Input: part model. Units: mm. Frame: model coordinates. A direction names the side the tool comes from. Give positions to 0.01 mm unless a question says otherwise; leave off trailing zeros. Loops run counter-clockwise (first coordinate to the right, second up) from the corner with the lowest first, then second, coordinate; pieces in that order, holes last. Notation, with made-up numbers: (52.5, 72) - (61.5, 72) arc R36 cw to (61.5, 111) - close; hole circle Ø10 at (-30.5, 20.25). An arc over 180 degrees is marked (long way). Answer as a JSON object with one key per item and string values. Group by question number.
(1) Material intervals for L1, parallel to X at y = -0.4, z = -3; L2, parallel to Y at x = 7.5, z = -7; L3, parallel to Z at x = -2, y = -4.8, sorted ascending.
(2) Section query D-D (z = -4.75). Return loops of the section in (x, y), plus the area to 3 significant figures.
(3) Mould query, pull axis X, two halves, no side actions, for faces 1 (the flat face through (11, -1, -6)), 2 (the flat face through (0, -4, -10)), 3 (the cylindrical face through (-5.55, -0.99, -1.57)). Classes: +X half, -X half, draft (parallel to the pull), parting line (faces both ways), or undercut.
(4) Pin query (flat end, axial travel): P1, Ø2, axis at x = -3, y = -2, coming from the -Z side; P2, Ø2.5, axis at x = 5, y = -4.5, coming from the +Z side; P3, Ø3.5, axis at x = 6, z = -3, coming from the -Y side. Return the tip coordinate at first contact, or that it passes through.
(5) Section query B-B (y = -1.7). Return loops of the section in (x, z), plus the area to 3 significant figures.
(6) Access query for faces 4 (the flat face through (0, -2, -5)), 5 (the cylindrical face through (6.45, -0.99, -1.57)). Directions: +Z, -Z, +X, -X, +Y, -Y. A direction counts if a zero-diameter tool reaches every point of the face in a straight line with its end or side. Return the directions, or none.
(7) Section query C-C (x = 5.75). Return loops of the section in (y, z).
(8) Section query A-A (x = -6). Return loops of the section in (y, z), plus the area to 3 significant figures.
```python
from build123d import *

# Parameters (mm, degrees)
SKETCH1_W                    = 12
SKETCH1_H                    = 2
BASE_FLANGE1_DEPTH           = 11
SKETCH2_R                    = 1.5
CUT_EXTRUDE1_DEPTH           = 10
EDGE_FLANGE1_STRIP_W         = 9.4732
EDGE_FLANGE1_STRIP_H         = 2
EDGE_FLANGE1_STRIP_CUT_DEPTH = 22
EDGE_FLANGE1_DEPTH           = 22


# Sheet-metal steps are written as plain solids
with BuildPart() as part:
    # Sketch1 → Base-Flange1 (new, symmetric)
    with BuildSketch(Plane(origin=(0, 0, 0), x_dir=(0, 0, -1), z_dir=(1, 0, 0))):
        with Locations((6, -1)):
            Rectangle(SKETCH1_W, SKETCH1_H)
    extrude(amount=BASE_FLANGE1_DEPTH, both=True)

    # Sketch2 → Cut-Extrude1 (cut)
    with BuildSketch(Plane(origin=(0, 0, 0), x_dir=(1, 0, 0), z_dir=(0, 1, 0))):
        with Locations(Location((-6, 3, 0), (0, 0, 270))):
            Circle(SKETCH2_R)
        with Locations(Location((6, 3, 0), (0, 0, 270))):
            Circle(SKETCH2_R)
    extrude(amount=-CUT_EXTRUDE1_DEPTH, mode=Mode.SUBTRACT)

    # Edge-Flange1 strip (across the edge) → Edge-Flange1 strip cut (cut)
    with BuildSketch(Plane(origin=(-11, -2, -12), x_dir=(0, 0, 1), z_dir=(1, 0, 0))):
        with Locations((-2, -1)):
            Rectangle(EDGE_FLANGE1_STRIP_W, EDGE_FLANGE1_STRIP_H)
    extrude(amount=EDGE_FLANGE1_STRIP_CUT_DEPTH, mode=Mode.SUBTRACT)

    # Edge-Flange1 section (across the edge) → Edge-Flange1 (add)
    with BuildSketch(Plane(origin=(-11, -2, -12), x_dir=(0, 0, 1), z_dir=(1, 0, 0))):
        with BuildLine():
            Line((0, 0.7366), (0, 3))
            Line((0, 3), (2, 3))
            Line((2, 3), (2, 0.7366))
            ThreePointArc((2, 0.7366), (2.215745145, 0.215745145), (2.7366, 0))
            Line((2.7366, 0), (2.7366, -2))
            ThreePointArc((2.7366, -2), (0.801531583, -1.198468417), (0, 0.7366))
        make_face()
    extrude(amount=EDGE_FLANGE1_DEPTH)


solid = part.part
```
Recorded:
{
 "1": {"L1": "x = -11 to -7.5, -4.5 to 4.5, 7.5 to 11", "L2": "y = -2 to 0", "L3": "z = -12 to -10"},
 "2": {"outline": "(-11, -2) - (11, -2) - (11, 0) - (-11, 0) - close", "area": "44.0 mm^2"},
 "3": {"face 1": "+X half", "face 2": "draft", "face 3": "undercut"},
 "4": {"P1": "stops at z = -12", "P2": "stops at z = -10", "P3": "stops at y = -2"},
 "5": {"outline": "(-11, -11.8) - (11, -11.8) - (11, 0) - (-11, 0) - close; hole circle Ø3 at (-6, -3); hole circle Ø3 at (6, -3)", "area": "245 mm^2"},
 "6": {"face 4": "+Z, +X, -X, -Y", "face 5": "+Y, -Y"},
 "7": {"outline": "(-5, -12) - (-2.74, -12) arc R2.74 ccw to (0, -9.26) - (0, -4.48) - (-2, -4.48) - (-2, -9.26) arc R0.74 cw to (-2.74, -10) - (-5, -10) - close; (-2, -1.52) - (0, -1.52) - (0, 0) - (-2, 0) - close"},
 "8": {"outline": "(-5, -12) - (-2.74, -12) arc R2.74 ccw to (0, -9.26) - (0, -4.5) - (-2, -4.5) - (-2, -9.26) arc R0.74 cw to (-2.74, -10) - (-5, -10) - close; (-2, -1.5) - (0, -1.5) - (0, 0) - (-2, 0) - close", "area": "22.5 mm^2"}
}
